from build123d import *

# Parameters (mm, degrees)
SKETCH_R     = 1
PAD_DEPTH    = 3
PAD001_DEPTH = 16.25
PAD002_DEPTH = 8
PAD003_DEPTH = 2


with BuildPart() as part:
    # Sketch → Pad (new body)
    with BuildSketch(Plane.YZ):
        Polygon((8.005182, 34), (8.005182, 41.5), (-10.5, 41.5), (-14, 35.310526), (-14, -35.310526), (-10.5, -41.5), (8.005182, -41.5), (8.005182, -34), (-10.5, -34), (-12, -32.5), (-12, 32.5), (-10.5, 34), align=None)
        with Locations((4.005182, 36.430913)):
            Circle(SKETCH_R, mode=Mode.SUBTRACT)
        with Locations((4.005182, -36.430913)):
            Circle(SKETCH_R, mode=Mode.SUBTRACT)
    pad = extrude(amount=-PAD_DEPTH)

    # Sketch002 (on Face15 of Pad) → Pad001 (join)
    with BuildSketch(Plane.YZ):
        Polygon((-10.5, 41.5), (8.005182, 41.5), (8.005182, 39.75), (-10.5, 39.75), (-12, 36.422085), (-12, -36.422085), (-10.5, -39.75), (8.005182, -39.75), (8.005182, -41.5), (-10.5, -41.5), (-14, -35.310526), (-14, 35.310526), align=None)
    pad001 = extrude(amount=PAD001_DEPTH)

    # Sketch003 (on Face6 of Pad001) → Pad002 (join)
    with BuildSketch(Plane(origin=(-3, 0, 0), x_dir=(0, 1, 0), z_dir=(-1, 0, 0))):
        Polygon((-12, 32.5), (-12, -32.5), (-10.5, -34), (-13.209125, -36.709125), (-14, -35.310526), (-14, 35.310526), (-13.209125, 36.709125), (-10.5, 34), align=None)
    pad002 = extrude(amount=PAD002_DEPTH)

    # Sketch004 (on Face28 of Pad002) → Pad003 (join)
    with BuildSketch(Plane(origin=(-11, 0, 0), x_dir=(0, 1, 0), z_dir=(-1, 0, 0))):
        Polygon((-6.041631, 40.085786), (-16.478994, 33.828846), (-13.655174, -33.40501), (-6.041631, -40.085786), (-1.926248, -35.970404), (-2.5, -33.829131), (-2.5, 33.829131), (-1.926248, 35.970404), align=None)
    pad003 = extrude(amount=-PAD003_DEPTH)

    # Mirrored: Pad, Pad001, Pad002, Pad003 across face of Pad003
    add(pad.mirror(Plane(origin=(16.25, -9.470165, 0), x_dir=(0, 1, 0), z_dir=(1, 0, 0))))
    add(pad001.mirror(Plane(origin=(16.25, -9.470165, 0), x_dir=(0, 1, 0), z_dir=(1, 0, 0))))
    add(pad002.mirror(Plane(origin=(16.25, -9.470165, 0), x_dir=(0, 1, 0), z_dir=(1, 0, 0))))
    add(pad003.mirror(Plane(origin=(16.25, -9.470165, 0), x_dir=(0, 1, 0), z_dir=(1, 0, 0))))


solid = part.part
Check sheet for the modelled part. Datum: model origin and axes. Units: mm. A direction names the side the tool comes from. Round coordinates to 2 decimals unless told otherwise and drop trailing zeros. Loops run counter-clockwise (first coordinate to the right, second up) from the corner with the lowest first, then second, coordinate; pieces in that order, holes last. Notation, with made-up numbers: M 89,45 L 124,45 A37 ccw 124,84 Z; hole C -18.75,50 d9. An arc over 180 degrees is marked long. One line per question, with ' | ' between items. Start each with the question number.
Item 1: Release check for a two-part mould opening along X. For faces 1 (the face through (34, -1, -34)), 2 (the face through (42.51, -2.22, -34.88)) record: released by +X, released by -X, zero draft, split by the parting line, or undercut.
Item 2: Section check C-C (x = 39). Record the boundary of the cut face in (y, z), and give its area (3 significant figures).
Item 3: Section check B-B (y = -7). Record the boundary of the cut face in (x, z).
Item 4: Section check D-D (z = 14). Record the boundary of the cut face in (x, y), and give its area (3 significant figures).
Item 5: Section check A-A (y = 6.5). Record the boundary of the cut face in (x, z).
Item 6: Set-up check for faces 3 (the face through (42.514, -4.013, 38.057)), 4 (the face through (42.514, -8.889, 37.587)), 5 (the face through (16, -1, 39.75)): record each of +Z, -Z, +X, -X, +Y, -Y from which the full face is reachable in a straight line by a thin tool's end or side.
Item 7: Gauge pin test, flat ends, axial feed: pin 1 Ø4 at (x, z) = (33, -20.5) entering from +Y; pin 2 Ø2 at (y, z) = (1, 37) entering from +X; pin 3 Ø2 at (x, z) = (-10.5, -15.5) entering from +Y. Record the tip position at first contact, or that the pin passes through.
Item 8: Scan lines: probe 1 along X at (y, z) = (-4.5, -37.5); probe 2 along X at (y, z) = (-4.25, -20); probe 3 along Z at (x, y) = (21, -8). Record each from-to range of solid material in increasing order.
Worked out:
1) face 1: undercut | face 2: zero draft
2) outline: M -14,-35.31 L -13.21,-36.71 L -10.5,-34 L -12,-32.5 L -12,32.5 L -10.5,34 L -13.21,36.71 L -14,35.31 Z | area: 149 mm^2
3) outline: M -11,-39.51 L -9,-39.51 L -9,39.24 L -11,39.24 Z; M -3,-41.5 L 35.5,-41.5 L 35.5,-34 L 32.5,-34 L 32.5,-39.75 L 0,-39.75 L 0,-34 L -3,-34 Z; M -3,34 L 0,34 L 0,39.75 L 32.5,39.75 L 32.5,34 L 35.5,34 L 35.5,41.5 L -3,41.5 Z; M 41.5,-39.51 L 43.5,-39.51 L 43.5,39.24 L 41.5,39.24 Z
4) outline: M -11,-14.47 L -9,-14.47 L -9,-14 L 41.5,-14 L 41.5,-14.47 L 43.5,-14.47 L 43.5,-2.5 L 41.5,-2.5 L 41.5,-12 L -9,-12 L -9,-2.5 L -11,-2.5 Z | area: 149 mm^2
5) outline: M -3,-41.5 L 35.5,-41.5 L 35.5,-34 L 32.5,-34 L 32.5,-39.75 L 0,-39.75 L 0,-34 L -3,-34 Z; M -3,34 L 0,34 L 0,39.75 L 32.5,39.75 L 32.5,34 L 35.5,34 L 35.5,41.5 L -3,41.5 Z
6) face 3: +Z, +X, +Y | face 4: +Z, +X | face 5: +Y
7) pin 1: y = -12 | pin 2: x = 35.5 | pin 3: y = -2.5
8) probe 1: -11 to -9, -3 to 0, 32.5 to 35.5, 41.5 to 43.5 | probe 2: -11 to -9, 41.5 to 43.5 | probe 3: -41.5 to -39.75, 39.75 to 41.5
